Geometry check sheet. Reference: the model listing, model coordinates, mm. Coordinates: 2 decimals unless noted, no trailing zeros. Loops run counter-clockwise (first coordinate to the right, second up) from the corner with the lowest first, then second, coordinate; pieces in that order, holes last.
Autodesk Inventor part; units mm, degrees
ref_plane "YZ Plane" through (0, 0, 0) normal (1, 0, 0) x (0, 1, 0)
ref_plane "XZ Plane" through (0, 0, 0) normal (0, 1, 0) x (-1, 0, 0)
ref_plane "XY Plane" through (0, 0, 0) normal (0, 0, 1) x (1, 0, 0)
sketch "Sketch1" plane through (0, 0, 0) normal (0, 1, 0) x (-1, 0, 0)
  line L0 (0, 0) -> (0, -315.198) construction
  line L1 (-4, 0) -> (-4, -315.198)
  line L2 (4, -315.198) -> (4, 0)
  arc A0 (4, 0) -> (-4, 0) centre (0, 0) ccw
  arc A1 (-4, -315.198) -> (4, -315.198) centre (0, -315.198) ccw
  circle A2 centre (0, 0) radius 1.5
  circle A3 centre (0, -315.198) radius 1.5
  arc A4 (-4, -3) -> (-4, -312.198) centre (780.9198, -157.599) ccw
  arc A5 (4, -3) -> (4, -312.198) centre (788.9198, -157.599) ccw
  point P0 (0, -157.599)
  dimension "d0" = 8
  dimension "d1" = 315.198
  dimension "d2" = 3
  dimension "d3" = 3
  dimension "d24" = 800
  dimension "d25" = 800
  dimension "d26" = 3
  dimension "d27" = 3
extrude "Extrusion1" add sketch "Sketch1" along normal blind 10 contours A0 L2 A5 L1 | L1 A5 A4 | L1 A5 L2 A1
sketch "Sketch4" plane through (0, 0, 0) normal (0, -1, 0) x (1, 0, 0)
  line L0 (-4, -315.198) -> (-4, -312.198)
  arc A0 (-4, -315.198) -> (4, -315.198) centre (0, -315.198) ccw
  line L1 (4, -312.198) -> (4, -315.198)
  arc A1 (4, -312.198) -> (4, -3) centre (-780.9198, -157.599) ccw
  line L2 (4, 0) -> (4, -3)
  arc A2 (4, 0) -> (-4, 0) centre (0, 0) ccw
  line L3 (-4, -3) -> (-4, 0)
  arc A3 (-4, -312.198) -> (-4, -3) centre (-788.9198, -157.599) ccw
  circle A4 centre (0, 0) radius 1.5
  circle A5 centre (0, -315.198) radius 1.5
  circle A6 centre (0, -315.198) radius 4
  point P0 (4, -315.198)
extrude "Extrusion3" add sketch "Sketch4" along normal blind 10 contours A6 A0
sketch "Sketch3" plane through (0, 10, 0) normal (0, 1, 0) x (1, 0, 0)
  line L0 (-4, 315.198) -> (-4, 312.198)
  arc A0 (-4, 3) -> (-4, 312.198) centre (-788.9198, 157.599) ccw
  line L1 (-4, 3) -> (-4, 0)
  arc A1 (-4, 0) -> (4, 0) centre (0, 0) ccw
  line L2 (4, 0) -> (4, 3)
  arc A2 (4, 3) -> (4, 312.198) centre (-780.9198, 157.599) ccw
  line L3 (4, 312.198) -> (4, 315.198)
  arc A3 (4, 315.198) -> (-4, 315.198) centre (0, 315.198) ccw
  circle A4 centre (0, 0) radius 1.5
  circle A5 centre (0, 315.198) radius 1.5
  arc A6 (-4, 3) -> (-4, 312.198) centre (-788.9198, 157.599) ccw
  line L4 (11.0802, 157.599) -> (14.7286, 165.8884)
  line L5 (14.7286, 165.8884) -> (19.0802, 157.599)
  arc A7 (4, 3) -> (4, 312.198) centre (-780.9198, 157.599) ccw
extrude "Extrusion2" [suppressed]
(1) Draft check along Z on faces 1 (the cylindrical face through (-0.521, -2.082, -319.164)), 2 (the cylindrical face through (0, 5, 4)), 3 (the cylindrical face through (11.077, 4.93, -159.777)), 4 (the flat face through (12, 10, -169)). Enter one of: +Z half, -Z half, draft (parallel to the pull), parting line (faces both ways), or undercut.
Findings:
face 1: parting line
face 2: +Z half
face 3: undercut
face 4: draft
(2) Gauge pin test, flat ends, axial feed: pin 1 Ø2.5 at (y, z) = (3, -1) entering from +X; pin 2 Ø3 at (x, y) = (2.5, 4.5) entering from +Z; pin 3 Ø10 at (y, z) = (-3, -238.5) entering from -X. Record the tip position at first contact, or that the pin passes through.
Findings:
pin 1: stops at x = 4
pin 2: stops at z = 3.87
pin 3: stops at x = 6.56
(3) Sectioned sample at A-A on y = 5. Record the cut outline in (x, z).
Findings:
outline: (-4, -315.2) arc R4 ccw to (4, -315.2) - (4, -312.2) arc R800 ccw to (4, -3) - (4, 0) arc R4 ccw to (-4, 0) - (-4, -3) arc R800 cw to (-4, -312.2) - close; hole circle Ø3 at (0, -315.2); hole circle Ø3 at (0, 0)
(4) Sectioned sample at B-B on y = -6.75. Record the cut outline in (x, z), and give its area (3 significant figures).
Findings:
outline: circle Ø8 at (0, -315.2); hole circle Ø3 at (0, -315.2)
area: 43.2 mm2
(5) Scan lines: L1, parallel to Z at x = 0, y = -3.75; L2, parallel to Y at x = 15.5, z = -116; L3, parallel to Z at x = 3.5, y = -4.75. Record each from-to range of solid material in increasing order.
Findings:
L1: z = -319.2 to -316.7, -313.7 to -311.2
L2: y = 0 to 10
L3: z = -317.13 to -313.26
(6) Sectioned sample at C-C on z = -284.5. Record the cut outline in (x, y), and give its area (3 significant figures).
Findings:
outline: (0.95, 0) - (8.95, 0) - (8.95, 10) - (0.95, 10) - close
area: 80.0 mm2
